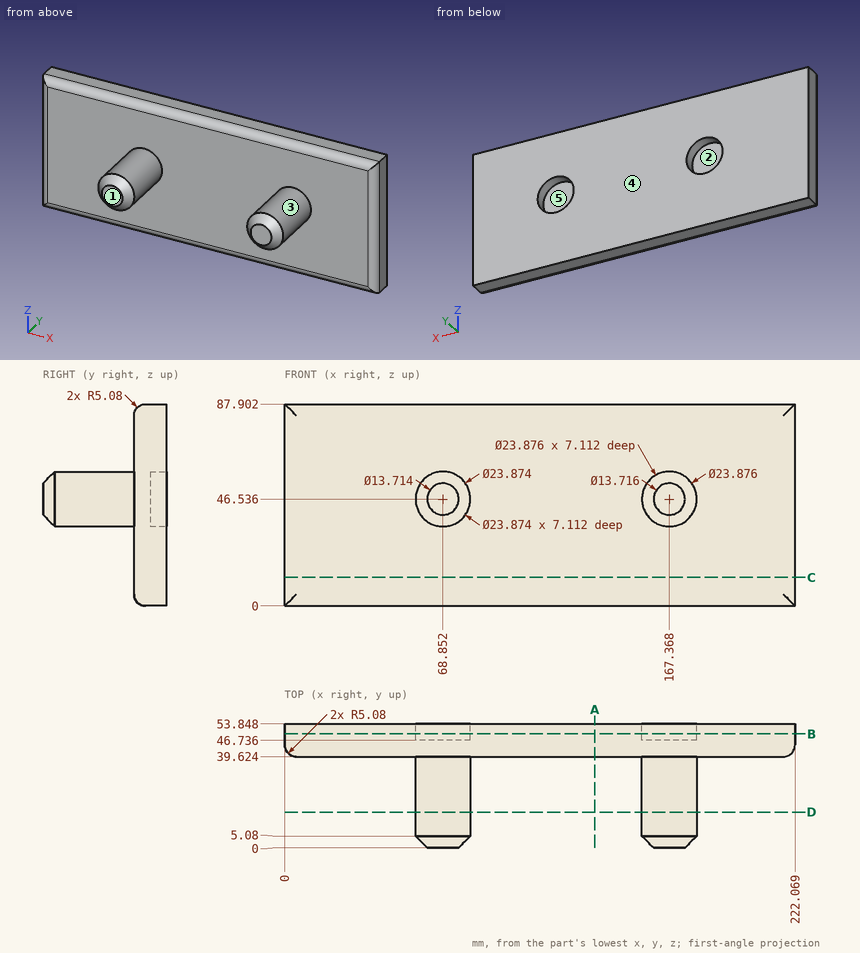
Job drawing, mm, ordinate dimensions from the low corner. One solid piece. A direction names the side the tool comes from. Round coordinates to 2 decimals unless told otherwise and drop trailing zeros. Write each loop counter-clockwise with the first axis right and the second up, starting at its lowest first coordinate (ties: lowest second). Pieces come first, ordered by that corner, then holes.
1) Band-saw the part on A-A, the plane x = 135. List the corners of the cut face in (y, z), and give its area (3 significant figures).
2) Pin check, flat tips, straight feed: pin 1 (12 mm diameter, centred on x = 180, z = 23, fed in from -Y); pin 2 (12 mm diameter, centred on y = 47.5, z = 55.5, fed in from -X); pin 3 (19 mm diameter, centred on x = 68.85, z = 46.54, fed in from +Y); pin 4 (3 mm diameter, centred on x = 141.5, y = 39, fed in from +Z) (1 decimal). Stop position of each tip, or through.
3) Band-saw the part on B-B, the plane y = 49.5. List the corners of the cut face in (x, z) (1 decimal), and give its area (3 significant figures).
4) Mould opens along X. For the marked faces 1 and 2 say: +X half, -X half, draft (parallel to the pull), parting line (faces both ways), or undercut.
5) 3-axis set-ups, long thin cutter, end or side, ignore diameter. For the marked faces 3, 4 and 5: which of +Z, -Z, +X, -X, +Y, -Y reach the whole face in a straight line?
6) Drill centre lines: probe 1 along Y at (x, z) = (61, 20.5); probe 2 along X at (y, z) = (44.5, 44.5) (1 decimal); probe 3 along X at (y, z) = (16, 38) (1 decimal). Where is each one in solid material? Low to high.
7) Band-saw the part on D-D, the plane y = 15.5. List the corners of the cut face in (x, z) (1 decimal).
8) Band-saw the part on C-C, the plane z = 12.5. List the corners of the cut face in (x, y), and give its area (3 significant figures).
Ans:
1. outline: (39.62, 5.08) arc R5.08 ccw to (44.7, 0) - (53.85, 0) - (53.85, 87.9) - (44.7, 87.9) arc R5.08 ccw to (39.62, 82.82) - close
1. area: 1,240 mm2
2. pin 1: stops at y = 39.62
2. pin 2: stops at x = 0
2. pin 3: stops at y = 46.74
2. pin 4: stops at z = 85.7
3. outline: (0, 0) - (222.1, 0) - (222.1, 87.9) - (0, 87.9) - close; hole circle Ø23.9 at (68.9, 46.5); hole circle Ø23.9 at (167.4, 46.5)
3. area: 18,600 mm2
4. face 1: draft
4. face 2: undercut
5. face 3: -Y
5. face 4: +Z, -Z, +X, -X, +Y
5. face 5: +Y
6. probe 1: y = 39.62 to 53.85
6. probe 2: x = 0 to 222.1
6. probe 3: x = 60.5 to 77.2, 159 to 175.7
7. outline: circle Ø23.9 at (68.9, 46.5); circle Ø23.9 at (167.4, 46.5)
8. outline: (0, 44.7) arc R5.08 ccw to (5.08, 39.62) - (216.99, 39.62) arc R5.08 ccw to (222.07, 44.7) - (222.07, 53.85) - (0, 53.85) - close
8. area: 3,150 mm2
